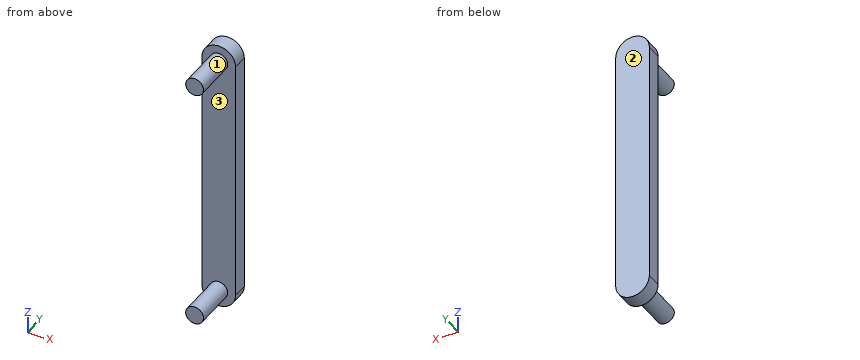
from build123d import *

# Parameters (mm, degrees)
SKETCH1_R             = 0.9
BOSS_EXTRUDE1_DEPTH   = 4.4
BOSS_EXTRUDE1_2_DEPTH = 4.4
BOSS_EXTRUDE2_DEPTH   = 1.5875


with BuildPart() as part:
    # Sketch1 → Boss-Extrude1 (new body)
    with BuildSketch(Plane(origin=(0, 0, 0), x_dir=(1, 0, 0), z_dir=(0, 1, 0))):
        with Locations(Location((0, 0, 0), (0, 0, 270))):
            Circle(SKETCH1_R)
    extrude(amount=BOSS_EXTRUDE1_DEPTH)



with BuildPart() as body_2:
    # Sketch1 → Boss-Extrude1 2 (new body)
    with BuildSketch(Plane(origin=(0, 0, 0), x_dir=(1, 0, 0), z_dir=(0, 1, 0))):
        with Locations(Location((0, -24.8, 0), (0, 0, 270))):
            Circle(SKETCH1_R)
    extrude(amount=BOSS_EXTRUDE1_2_DEPTH)


with BuildPart() as part_1:
    add(part.part)

    add(body_2.part)  # Boss-Extrude2 merges body 2
    # Sketch2 → Boss-Extrude2 (add)
    with BuildSketch(Plane(origin=(0, 4.4, 0), x_dir=(1, 0, 0), z_dir=(0, 1, 0))):
        with BuildLine():
            Line((1.7, 0), (1.7, -24.8))
            ThreePointArc((1.7, -24.8), (0, -26.5), (-1.7, -24.8))
            Line((-1.7, -24.8), (-1.7, 0))
            ThreePointArc((-1.7, 0), (0, 1.7), (1.7, 0))
        make_face()
    extrude(amount=BOSS_EXTRUDE2_DEPTH)


solid = part_1.part
Geometry check sheet. Reference: the model listing, model coordinates, mm. Face numbers are marked on the shaded views. Round coordinates to 2 decimals unless told otherwise and drop trailing zeros. Order: outer loops, then holes, each group sorted by start corner. A loop starts at its lowest first (then second) coordinate and runs counter-clockwise, first axis right, second up. Notation, with made-up numbers: (18, -19.5) -> (32, -19.5) arc R17 ccw to (32, -14.5) -> close; hole circle Ø6 at (46, 6). An arc over 180 degrees is marked (long way). Use one line per item in the form item = value.
1. Cross-section at C-C, the plane z = 8.25. Enter the section's corners in (x, y).
Working result:
outline = (-1.7, 4.4) -> (1.7, 4.4) -> (1.7, 5.99) -> (-1.7, 5.99) -> close
2. Cross-section at B-B, the plane x = 0. Enter the section's corners in (y, z).
Working result:
outline = (0, -0.9) -> (4.4, -0.9) -> (4.4, -1.7) -> (5.99, -1.7) -> (5.99, 26.5) -> (4.4, 26.5) -> (4.4, 25.7) -> (0, 25.7) -> (0, 23.9) -> (4.4, 23.9) -> (4.4, 0.9) -> (0, 0.9) -> close
3. Scan lines: line 1 along Y through (x, z) = (-0.85, 20); line 2 along Z through (x, y) = (0.8, 1.3); line 3 along Z through (x, y) = (-0.75, 0.9). Record each from-to range of solid material in increasing order. Write a range as from..to.
Working result:
line_1 = 4.4..5.99
line_2 = -0.41..0.41, 24.39..25.21
line_3 = -0.5..0.5, 24.3..25.3
4. Cross-section at A-A, the plane y = 0.85. Enter the section's corners in (x, z).
Working result:
outline = circle Ø1.8 at (0, 0); circle Ø1.8 at (0, 24.8)
5. Mould release check, pull along Z, two halves, no side actions. Record for the marked faces 1, 2 and 3: pulls with the +Z half, pulls with the -Z half, needs draft (parallel to the pull), parting line crosses it, or undercut.
Working result:
face_1 = undercut
face_2 = needs draft
face_3 = undercut
6. Cross-section at D-D, the plane y = 4.65. Enter the section's corners in (x, z), plus the area to 3 significant figures.
Working result:
outline = (-1.7, 0) arc R1.7 ccw to (1.7, 0) -> (1.7, 24.8) arc R1.7 ccw to (-1.7, 24.8) -> close
area = 93.4 mm^2
7. Go/stop test with flat-tipped pins: pin 1 (1.7 mm diameter, centred on x = 0, z = 12.5, fed in from -Y); pin 2 (1 mm diameter, centred on x = -0.5, y = 4.5, fed in from -Z); pin 3 (1.5 mm diameter, centred on x = -1, y = 3, fed in from -Z). Record where each tip stops, or that it passes through.
Working result:
pin_1 = 4.4
pin_2 = -1.7
pin_3 = -0.86
